Could you check a few things on this drawing? It's one solid part, dimensions in mm from its lowest x, y, z. A direction names the side the tool comes from. Give positions to 0.01 mm unless a question says otherwise; leave off trailing zeros. Write each loop counter-clockwise with the first axis right and the second up, starting at its lowest first coordinate (ties: lowest second). Pieces come first, ordered by that corner, then holes. Notation, with made-up numbers: (56, 86) - (113, 86) arc R25 ccw to (113, 105) - close; hole circle Ø10 at (50.25, -19.5). An arc over 180 degrees is marked (long way). One line per item, written item: value. Start each with the question number.
1) Imagine slicing it at A-A on x = 69. Write out the boundary of the cut face in (y, z) (1 decimal), plus the area to 3 significant figures.
2) We'd pull the mould along Z, two halves only. Please class the marked faces 5, 6 and 7: +Z half, -Z half, draft (parallel to the pull), parting line (faces both ways), or undercut.
3) On a 3-axis mill with a long thin cutter (end or side, diameter ignored), from which of +Z, -Z, +X, -X, +Y, -Y can I reach the whole of each face in a straight line? I mean the marked faces 1, 2, 3 and 4. Say none if no direction works.
4) Please list where these lines run through material, in increasing order: L1, parallel to Z at x = 11.5, y = 33; L2, parallel to Y at x = 39.5, z = 29. Write a range as [from, to].
5) Imagine slicing it at D-D on y = 7.5. Write out the boundary of the cut face in (x, z) (1 decimal), plus the area to 3 significant figures.
6) I'm going to push flat-ended pins straight in: P1, Ø14, axis at y = 57.5, z = 6, coming from the +X side; P2, Ø4, axis at x = 9.5, y = 65, coming from the -Z side; P3, Ø3.5, axis at y = 4, z = 34.5, coming from the +X side; P4, Ø6, axis at x = 63, z = 32.5, coming from the -Y side. Where does each tip first touch, or does it pass through?
7) Imagine slicing it at C-C on z = 6.35. Write out the boundary of the cut face in (x, y).
8) Imagine slicing it at B-B on y = 30. Write out the boundary of the cut face in (x, z).
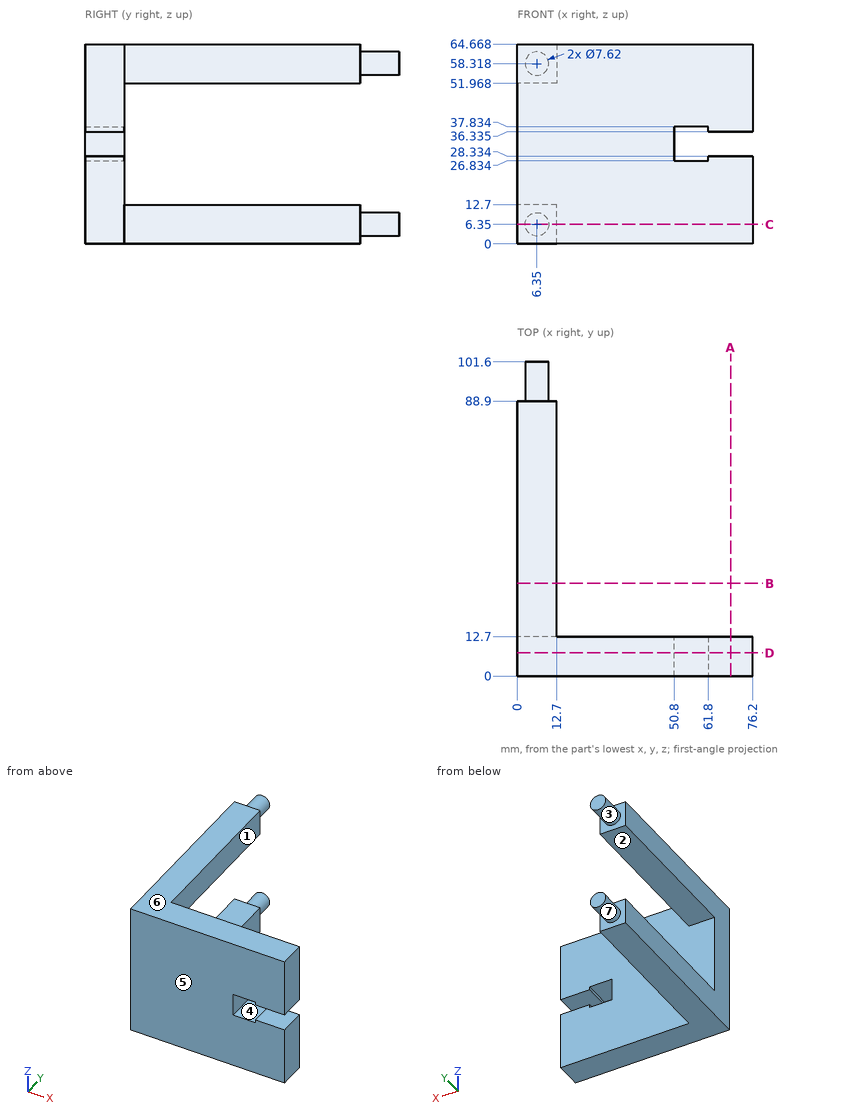
Numbers:
1. outline: (0, 0) - (12.7, 0) - (12.7, 28.3) - (0, 28.3) - close; (0, 36.3) - (12.7, 36.3) - (12.7, 64.7) - (0, 64.7) - close
1. area: 720 mm^2
2. face 5: draft
2. face 6: +Z half
2. face 7: undercut
3. face 1: +Z, -Z, +X, +Y
3. face 2: +X, -X, +Y
3. face 3: +Y
3. face 4: +Y, -Y
4. L1: [0, 12.7], [51.97, 64.67]
4. L2: [0, 12.7]
5. outline: (0, 0) - (76.2, 0) - (76.2, 28.3) - (61.8, 28.3) - (61.8, 26.8) - (50.8, 26.8) - (50.8, 37.8) - (61.8, 37.8) - (61.8, 36.3) - (76.2, 36.3) - (76.2, 64.7) - (0, 64.7) - close
5. area: 4,690 mm^2
6. P1: x = 12.7
6. P2: z = 0
6. P3: x = 50.8
6. P4: through
7. outline: (0, 0) - (76.2, 0) - (76.2, 12.7) - (12.7, 12.7) - (12.7, 88.9) - (10.16, 88.9) - (10.16, 101.6) - (2.54, 101.6) - (2.54, 88.9) - (0, 88.9) - close
8. outline: (0, 0) - (12.7, 0) - (12.7, 12.7) - (0, 12.7) - close; (0, 51.97) - (12.7, 51.97) - (12.7, 64.67) - (0, 64.67) - close
